```python
from build123d import *

# Parameters (mm, degrees)
ESBO_O1_R                  = 3.35
RESSALTO_EXTRUS_O1_DEPTH   = 2.2
ESBO_O2_W                  = 25
ESBO_O2_H                  = 2.2
RESSALTO_EXTRUS_O2_DEPTH   = 21.8
CORTE_EXTRUS_O2_DEPTH      = 40.687277558
CORTE_EXTRUS_O2_DEPTH_BACK = 24
ESBO_O3_R                  = 2.5
FILETE1_R                  = 1


with BuildPart() as part:
    # Esboço1 → Ressalto-extrusão1 (new body)
    with BuildSketch(Plane.XY):
        with BuildLine():
            ThreePointArc((19.671946284, -6.495902042), (15.467093732, -9.437851933), (12.5, -13.625))
            Line((12.5, -13.625), (-12.5, -13.625))
            ThreePointArc((-12.5, -13.625), (-15.467093732, -9.437851933), (-19.671946284, -6.495902042))
            ThreePointArc((-19.671946284, -6.495902042), (-23.628167932, 1.560853588), (-16.625, 7.175))
            Line((-16.625, 7.175), (16.625, 7.175))
            ThreePointArc((16.625, 7.175), (23.628167932, 1.560853588), (19.671946284, -6.495902042))
        make_face()
        with Locations((16.625, 0)):
            Circle(ESBO_O1_R, mode=Mode.SUBTRACT)
        with Locations((-16.625, 0)):
            Circle(ESBO_O1_R, mode=Mode.SUBTRACT)
    extrude(amount=RESSALTO_EXTRUS_O1_DEPTH)

    # Esboço2 → Ressalto-extrusão2 (add)
    with BuildSketch(Plane.XY.offset(2.2)):
        with Locations((0, -12.525)):
            Rectangle(ESBO_O2_W, ESBO_O2_H)
    extrude(amount=RESSALTO_EXTRUS_O2_DEPTH)

    # Esboço3 → Corte-extrusão2 (cut, two sides: drawn at the far end of the back side and taken through both)
    with BuildSketch(Plane.XZ.offset(13.625).offset(-CORTE_EXTRUS_O2_DEPTH_BACK)):
        with Locations(Location((0, 16.8, 0), (0, 0, 90))):
            Circle(ESBO_O3_R)
        with BuildLine():
            ThreePointArc((-12.5, 2.2), (-8.565992578, 9.033887716), (-7.2, 16.8))
            ThreePointArc((-7.2, 16.8), (-5.091168815, 21.891168834), (2.7e-08, 24))
            Line((2.7e-08, 24), (-12.5, 24))
            Line((-12.5, 24), (-12.5, 2.2))
        make_face()
        with BuildLine():
            Line((12.5, 24), (2.7e-08, 24))
            ThreePointArc((2.7e-08, 24), (5.091168834, 21.891168815), (7.2, 16.8))
            ThreePointArc((7.2, 16.8), (8.565992578, 9.033887716), (12.5, 2.2))
            Line((12.5, 2.2), (12.5, 24))
        make_face()
    extrude(amount=CORTE_EXTRUS_O2_DEPTH + CORTE_EXTRUS_O2_DEPTH_BACK, mode=Mode.SUBTRACT)

    # Filete1
    filete1_edges = [part.edges().sort_by_distance(p)[0] for p in [
        (12.5, -12.525, 2.2),
        (-12.5, -12.525, 2.2),
        (0, -11.425, 2.2),
    ]]
    fillet(filete1_edges, radius=FILETE1_R)
    filete1_2_edges = [part.edges().sort_by_distance(p)[0] for p in [
        (0, -13.625, 0),
        (12.5, -13.625, 1.159674218),
        (-12.5, -13.625, 1.159674218),
    ]]
    fillet(filete1_2_edges, radius=FILETE1_R)


solid = part.part
```
Verification items for the finished model (mm, model axes). A direction names the side the tool comes from. Give positions to 0.01 mm unless a question says otherwise; leave off trailing zeros. Loops run counter-clockwise (first coordinate to the right, second up) from the corner with the lowest first, then second, coordinate; pieces in that order, holes last.
1. Section check D-D, the plane z = 7.75. Enter the section's corners in (x, y) (3 decimals), then the cut area to 3 significant figures.
2. Thickness scan on line 1 (Z direction, x = -8, y = 2); line 2 (Y direction, x = 1, z = 7.5) (3 decimals). Record the ranges inside material, lowest first.
3. Section check C-C, the plane x = 3. Enter the section's corners in (y, z) (3 decimals).
4. Section check B-B, the plane z = 15.75. Enter the section's corners in (x, y) (3 decimals).
5. Section check A-A, the plane y = 0. Enter the section's corners in (x, z) (3 decimals), then the cut area to 3 significant figures.
6. Go/stop test with flat-tipped pins: pin 1 Ø6 at (x, y) = (16.625, 0) entering from -Z; pin 2 Ø3 at (x, z) = (-0.5, 14) entering from +Y (3 decimals); pin 3 Ø4 at (y, z) = (-11.5, 15) entering from +X; pin 4 Ø7.5 at (x, y) = (-16.625, 0) entering from +Z. Record where each tip stops, or that it passes through.
7. Set-up check for faces 1 (the flat face through (0, 7.175, 1)), 2 (the flat face through (0, -11.425, 11)): record each of +Z, -Z, +X, -X, +Y, -Y from which the full face is reachable in a straight line by a thin tool's end or side.
8. Mould release check, pull along X, two halves, no side actions. Record for faces 3 (the flat face through (0, -3, 0)), 4 (the cylindrical face through (13.28, 0.15, 1.08)), 5 (the cylindrical face through (-23.656, 1.428, 1.085)): released by +X, released by -X, zero draft, split by the parting line, or undercut.
Geometry says:
1. outline: (-9.077, -13.625) - (9.077, -13.625) - (9.077, -11.425) - (-9.077, -11.425) - close
1. area: 39.9 mm2
2. line 1: z = 0 to 2.2
2. line 2: y = -13.625 to -11.425
3. outline: (-13.625, 1) arc R1 ccw to (-12.625, 0) - (7.175, 0) - (7.175, 2.2) - (-10.425, 2.2) arc R1 cw to (-11.425, 3.2) - (-11.425, 23.345) - (-13.625, 23.345) - close
4. outline: (-7.224, -13.625) - (-2.269, -13.625) - (-2.269, -11.425) - (-7.224, -11.425) - close; (2.269, -13.625) - (7.224, -13.625) - (7.224, -11.425) - (2.269, -11.425) - close
5. outline: (-23.8, 0) - (-19.975, 0) - (-19.975, 2.2) - (-23.8, 2.2) - close; (-13.275, 0) - (13.275, 0) - (13.275, 2.2) - (-13.275, 2.2) - close; (19.975, 0) - (23.8, 0) - (23.8, 2.2) - (19.975, 2.2) - close
5. area: 75.2 mm2
6. pin 1: passes through
6. pin 2: stops at y = -11.425
6. pin 3: stops at x = 7.52
6. pin 4: stops at z = 2.2
7. face 1: +Z, -Z, +X, -X, +Y
7. face 2: +Z, +X, -X, +Y
8. face 3: zero draft
8. face 4: undercut
8. face 5: released by -X
